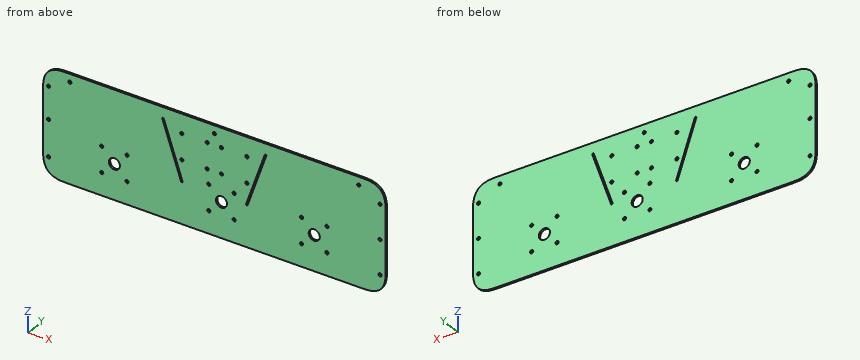
```python
from build123d import *

# Parameters (mm, degrees)
SKETCH1_W           = 432
SKETCH1_H           = 200
BOSS_EXTRUDE1_DEPTH = 2.5
SKETCH3_R           = 7
SKETCH3_R_2         = 2
SKETCH3_W           = 498.20945101
SKETCH3_H           = 57.36356312
CUT_EXTRUDE1_DEPTH  = 2.5
SKETCH5_W           = 366.875294571
SKETCH5_H           = 10
SKETCH5_W_2         = 65.124705429
CUT_EXTRUDE3_DEPTH  = 2.5
SKETCH6_R           = 2
CUT_EXTRUDE4_DEPTH  = 2.5
CUT_EXTRUDE5_DEPTH  = 2.5
FILLET1_SIZE        = 30
SKETCH9_R           = 2
CUT_EXTRUDE6_DEPTH  = 2.5
SKETCH10_R          = 2
CUT_EXTRUDE7_DEPTH  = 2.5
SKETCH11_R          = 7
SKETCH11_R_2        = 2
CUT_EXTRUDE8_DEPTH  = 10


with BuildPart() as part:
    # Sketch1 → Boss-Extrude1 (new body)
    with BuildSketch(Plane(origin=(0, 0, 0), x_dir=(1, 0, 0), z_dir=(0, 1, 0))):
        with Locations((112.865968756, 71.914913526)):
            Rectangle(SKETCH1_W, SKETCH1_H)
    extrude(amount=BOSS_EXTRUDE1_DEPTH)

    # Sketch3 → Cut-Extrude1 (cut)
    with BuildSketch(Plane(origin=(0, 2.5, 0), x_dir=(1, 0, 0), z_dir=(0, 1, 0))):
        with Locations(Location((-13.134031244, 71.914913526, 0), (0, 0, 270))):
            Circle(SKETCH3_R)
        with Locations(Location((-29.135857702, 55.913087067, 0), (0, 0, 270))):
            Circle(SKETCH3_R_2)
        with Locations(Location((-29.135857702, 87.916739984, 0), (0, 0, 270))):
            Circle(SKETCH3_R_2)
        with Locations(Location((2.867795214, 55.913087067, 0), (0, 0, 270))):
            Circle(SKETCH3_R_2)
        with Locations(Location((2.867795214, 87.916739984, 0), (0, 0, 270))):
            Circle(SKETCH3_R_2)
        with Locations(Location((238.865968756, 71.914913526, 0), (0, 0, 270))):
            Circle(SKETCH3_R)
        with Locations((79.761243251, 144.596695086)):
            Rectangle(SKETCH3_W, SKETCH3_H)
        with Locations(Location((222.864142298, 55.913087067, 0), (0, 0, 270))):
            Circle(SKETCH3_R_2)
        with Locations(Location((254.867795214, 87.916739984, 0), (0, 0, 270))):
            Circle(SKETCH3_R_2)
        with Locations(Location((222.864142298, 87.916739984, 0), (0, 0, 270))):
            Circle(SKETCH3_R_2)
        with Locations(Location((254.867795214, 55.913087067, 0), (0, 0, 270))):
            Circle(SKETCH3_R_2)
    extrude(amount=-CUT_EXTRUDE1_DEPTH, mode=Mode.SUBTRACT)

    # Sketch5 → Cut-Extrude3 (cut)
    with BuildSketch(Plane(origin=(0, 2.5, 0), x_dir=(1, 0, 0), z_dir=(0, 1, 0))):
        with Locations((80.303616041, -23.085086474)):
            Rectangle(SKETCH5_W, SKETCH5_H)
        with Locations((296.303616042, -23.085086474)):
            Rectangle(SKETCH5_W_2, SKETCH5_H)
    extrude(amount=-CUT_EXTRUDE3_DEPTH, mode=Mode.SUBTRACT)

    # Sketch6 → Cut-Extrude4 (cut)
    with BuildSketch(Plane(origin=(0, 2.5, 0), x_dir=(1, 0, 0), z_dir=(0, 1, 0))):
        with Locations(Location((71.864142298, 5.913087067, 0), (0, 0, 270))):
            Circle(SKETCH6_R)
        with Locations(Location((71.864142298, 37.916739984, 0), (0, 0, 270))):
            Circle(SKETCH6_R)
        with Locations(Location((103.867795214, 37.916739984, 0), (0, 0, 270))):
            Circle(SKETCH6_R)
        with Locations(Location((103.867795214, 5.913087067, 0), (0, 0, 270))):
            Circle(SKETCH6_R)
        with Locations(Location((121.864142298, 5.913087067, 0), (0, 0, 270))):
            Circle(SKETCH6_R)
        with Locations(Location((121.864142298, 37.916739984, 0), (0, 0, 270))):
            Circle(SKETCH6_R)
        with Locations(Location((153.867795214, 37.916739984, 0), (0, 0, 270))):
            Circle(SKETCH6_R)
        with Locations(Location((153.867795214, 5.913087067, 0), (0, 0, 270))):
            Circle(SKETCH6_R)
    extrude(amount=-CUT_EXTRUDE4_DEPTH, mode=Mode.SUBTRACT)

    # Sketch8 → Cut-Extrude5 (cut)
    with BuildSketch(Plane(origin=(0, 2.5, 0), x_dir=(1, 0, 0), z_dir=(0, 1, 0))):
        with BuildLine():
            Line((176.582305496, -4.412929011), (152.923062834, 63.765083659))
            ThreePointArc((152.923062834, 63.765083659), (153.539952677, 65.037658577), (154.812527595, 64.420768733))
            Line((154.812527595, 64.420768733), (178.471770257, -3.757243937))
            ThreePointArc((178.471770257, -3.757243937), (177.854880414, -5.029818855), (176.582305496, -4.412929011))
        make_face()
        with BuildLine():
            Line((47.260167255, -3.757243937), (70.919409917, 64.420768733))
            ThreePointArc((70.919409917, 64.420768733), (72.191984835, 65.037658577), (72.808874679, 63.765083659))
            Line((72.808874679, 63.765083659), (49.149632016, -4.412929011))
            ThreePointArc((49.149632016, -4.412929011), (47.877057099, -5.029818855), (47.260167255, -3.757243937))
        make_face()
    extrude(amount=-CUT_EXTRUDE5_DEPTH, mode=Mode.SUBTRACT)

    # Fillet1
    # a fillet whose section is not a circle: 30 mm, written as the material it takes off along each edge
    with BuildSketch(Plane(origin=(-103.134031244, -75, -115.914913526), x_dir=(0, 0, 1), z_dir=(0, 1, 0)), Plane(origin=(-103.134031244, 77.5, 18.085086474), x_dir=(0, 0, -1), z_dir=(0, -1, 0)), Plane(origin=(328.865968756, 77.5, 18.085086474), x_dir=(-1, 0, 0), z_dir=(0, -1, 0))) as fillet1_piece_1:
        with BuildLine():
            add(Edge.make_bspline([(FILLET1_SIZE, 0), (FILLET1_SIZE * 0.831801948466, 0), (FILLET1_SIZE * 0.663603896932, 0), (FILLET1_SIZE * 0.292893218813, FILLET1_SIZE * 0.0716919198361), (FILLET1_SIZE * 0.0716919198361, FILLET1_SIZE * 0.292893218813), (0, FILLET1_SIZE * 0.663603896932), (0, FILLET1_SIZE * 0.831801948466), (0, FILLET1_SIZE)], knots=[0, 0, 0, 0, 0, 0, 0.5, 0.5, 1, 1, 1, 1, 1, 1], degree=5))
            Line((0, FILLET1_SIZE), (0, 0))
            Line((0, 0), (FILLET1_SIZE, 0))
        make_face()
    extrude(amount=152.5, mode=Mode.SUBTRACT)
    with BuildSketch(Plane(origin=(328.865968756, 77.5, -115.914913526), x_dir=(-1, 0, 0), z_dir=(0, -1, 0))) as fillet1_piece_2:
        with BuildLine():
            add(Edge.make_bspline([(FILLET1_SIZE, 0), (FILLET1_SIZE * 0.831801948466, 0), (FILLET1_SIZE * 0.663603896932, 0), (FILLET1_SIZE * 0.292893218813, -FILLET1_SIZE * 0.0716919198361), (FILLET1_SIZE * 0.0716919198361, -FILLET1_SIZE * 0.292893218813), (0, -FILLET1_SIZE * 0.663603896932), (0, -FILLET1_SIZE * 0.831801948466), (0, -FILLET1_SIZE)], knots=[0, 0, 0, 0, 0, 0, 0.5, 0.5, 1, 1, 1, 1, 1, 1], degree=5))
            Line((0, -FILLET1_SIZE), (0, 0))
            Line((0, 0), (FILLET1_SIZE, 0))
        make_face()
    extrude(amount=152.5, mode=Mode.SUBTRACT)

    # Sketch9 → Cut-Extrude6 (cut)
    with BuildSketch(Plane(origin=(0, 2.5, 0), x_dir=(1, 0, 0), z_dir=(0, 1, 0))):
        with Locations(Location((321.865968752, 6.010283068, 0), (0, 0, 270))):
            Circle(SKETCH9_R)
        with Locations(Location((321.865968752, 48.914945481, 0), (0, 0, 270))):
            Circle(SKETCH9_R)
        with Locations(Location((321.865968752, 91.819607898, 0), (0, 0, 270))):
            Circle(SKETCH9_R)
        with Locations(Location((-96.134031244, 46.467317494, 0), (0, 0, 270))):
            Circle(SKETCH9_R)
        with Locations(Location((-96.134031244, 91.819607898, 0), (0, 0, 270))):
            Circle(SKETCH9_R)
        with Locations(Location((-96.134031244, 6.010283068, 0), (0, 0, 270))):
            Circle(SKETCH9_R)
    extrude(amount=-CUT_EXTRUDE6_DEPTH, mode=Mode.SUBTRACT)

    # Sketch10 → Cut-Extrude7 (cut)
    with BuildSketch(Plane(origin=(0, 2.5, 0), x_dir=(1, 0, 0), z_dir=(0, 1, 0))):
        with Locations(Location((112.866022655, -8.085086472, 0), (0, 0, 270))):
            Circle(SKETCH10_R)
        with Locations(Location((294.941757967, -8.085086472, 0), (0, 0, 270))):
            Circle(SKETCH10_R)
        with Locations(Location((-69.209712656, -8.085086472, 0), (0, 0, 270))):
            Circle(SKETCH10_R)
    extrude(amount=-CUT_EXTRUDE7_DEPTH, mode=Mode.SUBTRACT)

    # Sketch11 → Cut-Extrude8 (cut)
    with BuildSketch(Plane(origin=(0, 2.5, 0), x_dir=(1, 0, 0), z_dir=(0, 1, 0))):
        with Locations(Location((121.864142298, 71.914913526, 0), (0, 0, 270))):
            Circle(SKETCH11_R)
        with Locations(Location((105.86231584, 55.913087067, 0), (0, 0, 270))):
            Circle(SKETCH11_R_2)
        with Locations(Location((137.865968756, 87.916739984, 0), (0, 0, 270))):
            Circle(SKETCH11_R_2)
        with Locations(Location((137.865968756, 55.913087067, 0), (0, 0, 270))):
            Circle(SKETCH11_R_2)
        with Locations(Location((105.86231584, 87.916739984, 0), (0, 0, 270))):
            Circle(SKETCH11_R_2)
    extrude(amount=-CUT_EXTRUDE8_DEPTH, mode=Mode.SUBTRACT)


solid = part.part
```
Read the model definition and answer for the solid it produces. Units are mm, in the model's axes. Give positions to 0.01 mm unless a question says otherwise; leave off trailing zeros. Order: outer loops, then holes, each group sorted by start corner. A loop starts at its lowest first (then second) coordinate and runs counter-clockwise, first axis right, second up.
(1) Find section B-B (y = 1.4). Give the number of separate pieces and of enclosed holes in the cut face, plus the area to 3 significant figures.
(2) Straight lines are drawn through the part: L1, parallel to X at y = 0.65, z = -71.5; L2, parallel to X at y = 0.9, z = 1; L3, parallel to X at y = 0.1, z = -62. For each, find the intervals that lie inside material, in ascending order.
(3) Given pin 1 (2.5 mm diameter, centred on x = 254.87, z = -55.91, fed in from +Y), flat-ended and moving along its own axis, determine where the tip first touches the part or whether it passes through.
(4) Find section A-A (z = -71.5). Give the vertices of the cut face in (x, y), plus the area to 3 significant figures.
Result sheet:
1. separate pieces: 1
1. enclosed holes: 34
1. area: 56,300 mm2
2. L1: x = -103.13 to -20.12, -6.15 to 114.88, 128.85 to 231.88, 245.85 to 328.87
2. L2: x = -102.03 to 48.22, 50.33 to 175.4, 177.51 to 327.76
2. L3: x = -103.13 to 70.08, 72.2 to 153.54, 155.65 to 328.87
3. pin 1: passes through
4. outline: (-103.13, 0) - (-20.12, 0) - (-20.12, 2.5) - (-103.13, 2.5) - close; (-6.15, 0) - (114.88, 0) - (114.88, 2.5) - (-6.15, 2.5) - close; (128.85, 0) - (231.88, 0) - (231.88, 2.5) - (128.85, 2.5) - close; (245.85, 0) - (328.87, 0) - (328.87, 2.5) - (245.85, 2.5) - close
4. area: 975 mm2
